```python
from build123d import *

# Parameters (mm, degrees)
SKETCH1_W                    = 124.750351958
SKETCH1_H                    = 19.070117496
BASE_FLANGE1_DEPTH           = 6
EDGE_FLANGE1_STRIP_W         = 26
EDGE_FLANGE1_STRIP_H         = 6
EDGE_FLANGE1_STRIP_CUT_DEPTH = 19.070117497
EDGE_FLANGE1_DEPTH           = 19.070117497
EDGE_FLANGE2_STRIP_W         = 26
EDGE_FLANGE2_STRIP_H         = 6
EDGE_FLANGE2_STRIP_CUT_DEPTH = 19.070117497
EDGE_FLANGE2_DEPTH           = 19.070117497


# Sheet-metal steps are written as plain solids
with BuildPart() as part:
    # Sketch1 → Base-Flange1 (new body)
    with BuildSketch(Plane(origin=(0, 0, 0), x_dir=(0, 0, -1), z_dir=(1, 0, 0))):
        Rectangle(SKETCH1_W, SKETCH1_H)
    extrude(amount=-BASE_FLANGE1_DEPTH)

    # Edge-Flange1 strip (across the edge) → Edge-Flange1 strip cut (cut)
    with BuildSketch(Plane(origin=(0, 9.535058748, 62.375175979), x_dir=(0, 0, -1), z_dir=(0, -1, 0))):
        with Locations((-6, -3)):
            Rectangle(EDGE_FLANGE1_STRIP_W, EDGE_FLANGE1_STRIP_H)
    extrude(amount=EDGE_FLANGE1_STRIP_CUT_DEPTH, mode=Mode.SUBTRACT)

    # Edge-Flange1 section (across the edge) → Edge-Flange1 (add)
    with BuildSketch(Plane(origin=(0, 9.535058748, 62.375175979), x_dir=(0, 0, -1), z_dir=(0, -1, 0))):
        with BuildLine():
            Line((0, 1), (0, 94))
            Line((0, 94), (6, 94))
            Line((6, 94), (6, 1))
            ThreePointArc((6, 1), (6.292893219, 0.292893219), (7, 0))
            Line((7, 0), (7, -6))
            ThreePointArc((7, -6), (2.050252532, -3.949747468), (0, 1))
        make_face()
    extrude(amount=EDGE_FLANGE1_DEPTH)

    # Edge-Flange2 strip (across the edge) → Edge-Flange2 strip cut (cut)
    with BuildSketch(Plane(origin=(94, -9.535058748, 62.375175979), x_dir=(-1, 0, 0), z_dir=(0, 1, 0))):
        with Locations((-6, -3)):
            Rectangle(EDGE_FLANGE2_STRIP_W, EDGE_FLANGE2_STRIP_H)
    extrude(amount=EDGE_FLANGE2_STRIP_CUT_DEPTH, mode=Mode.SUBTRACT)

    # Edge-Flange2 section (across the edge) → Edge-Flange2 (add)
    with BuildSketch(Plane(origin=(94, -9.535058748, 62.375175979), x_dir=(-1, 0, 0), z_dir=(0, 1, 0))):
        with BuildLine():
            Line((0, 1), (0, 144))
            Line((0, 144), (6, 144))
            Line((6, 144), (6, 1))
            ThreePointArc((6, 1), (6.292893219, 0.292893219), (7, 0))
            Line((7, 0), (7, -6))
            ThreePointArc((7, -6), (2.050252532, -3.949747468), (0, 1))
        make_face()
    extrude(amount=EDGE_FLANGE2_DEPTH)


solid = part.part
```
For this review, take the finished solid that the model builds, in its own axes (mm). A direction names the side the tool comes from. Give positions to 0.01 mm unless a question says otherwise; leave off trailing zeros. Write each loop counter-clockwise with the first axis right and the second up, starting at its lowest first coordinate (ties: lowest second). Pieces come first, ordered by that corner, then holes.
Item 1: Wall thickness on probe 1 along X at (y, z) = (-7.75, -28.5); probe 2 along Z at (x, y) = (41, -2.25); probe 3 along X at (y, z) = (-7.5, 75): over which ranges is each line inside the solid? List them lowest first.
Item 2: Take a section at C-C (z = 69). Give the boundary of the cut face in (x, y), and give its area (3 significant figures).
Item 3: Take a section at A-A (y = 2). Give the boundary of the cut face in (x, z), and give its area (3 significant figures).
Item 4: Machinability: for faces 1 (the face through (45, 0, 56.375)), 2 (the face through (43, 0, 62.375)), 3 (the face through (94, 0, 134)), which of the approach directions +Z, -Z, +X, -X, +Y, -Y give a long, thin tool a straight path to every point of the face, cutting with its end or side? Answer none if there is none.
Item 5: Insertion check: P1, Ø3, axis at x = 58, y = 4, coming from the -Z side; P2, Ø5.5, axis at x = 37, y = -1, coming from the +Z side; P3, Ø2, axis at y = -3.5, z = 58.5, coming from the +X side. Each pin has a flat end and moves straight along its axis. Give the tip position at first contact, or say it passes through.
Item 6: Take a section at B-B (x = 22). Give the boundary of the cut face in (y, z), and give its area (3 significant figures).
Established:
1. probe 1: x = -6 to 0
1. probe 2: z = 56.38 to 62.38
1. probe 3: x = 88 to 94
2. outline: (88, -9.54) - (94, -9.54) - (94, 9.54) - (88, 9.54) - close
2. area: 114 mm2
3. outline: (-6, -62.38) - (0, -62.38) - (0, 55.38) arc R1 cw to (1, 56.38) - (87, 56.38) arc R7 ccw to (94, 63.38) - (94, 206.38) - (88, 206.38) - (88, 63.38) arc R1 cw to (87, 62.38) - (1, 62.38) arc R7 ccw to (-6, 55.38) - close
3. area: 2,160 mm2
4. face 1: -Z, +X, +Y, -Y
4. face 2: +Z, -X, +Y, -Y
4. face 3: +Z, -Z, +X, +Y, -Y
5. P1: stops at z = 56.38
5. P2: stops at z = 62.38
5. P3: stops at x = 92.83
6. outline: (-9.54, 56.38) - (9.54, 56.38) - (9.54, 62.38) - (-9.54, 62.38) - close
6. area: 114 mm2
